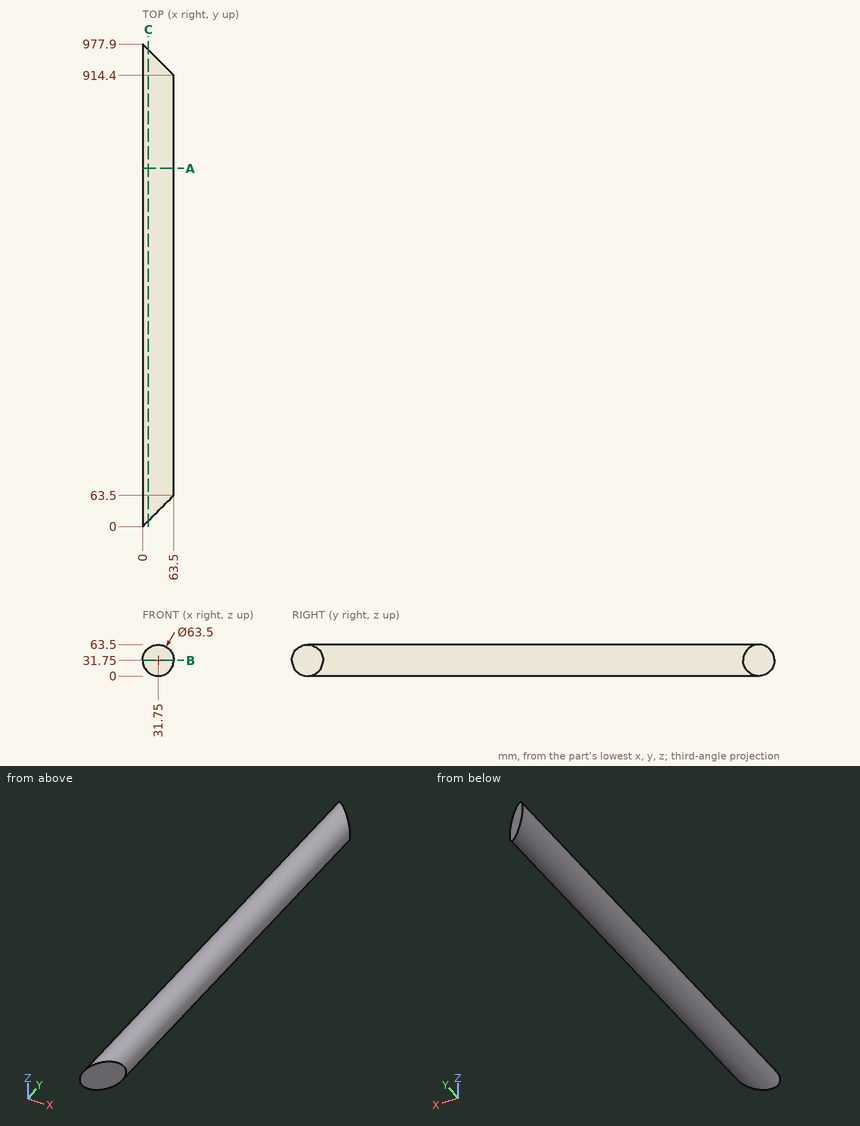
Can you work these out from the drawing? Everything is in mm from the part's minimum corner. Round coordinates to 2 decimals unless told otherwise and drop trailing zeros. Loops run counter-clockwise (first coordinate to the right, second up) from the corner with the lowest first, then second, coordinate; pieces in that order, holes last. Notation, with made-up numbers: (11, -26) - (62, -26) arc R6 ccw to (62, -19) - close; hole circle Ø7 at (75.5, -20). An arc over 180 degrees is marked (long way). One line per question, with ' | ' between items. Start each with the question number.
Q1. I want a section at C-C (x = 12). Write out the boundary of the cut face in (y, z).
Q2. I want a section at B-B (z = 31.75). Write out the boundary of the cut face in (x, y), then the cut area to 3 significant figures.
Q3. Will these pins go through, and if not, where does the flat tip stop? pin 1 (6 mm diameter, centred on x = 16, y = 178, fed in from -Z); pin 2 (8 mm diameter, centred on x = 12, y = 551, fed in from -Z); pin 3 (1 mm diameter, centred on x = 27.5, y = 336, fed in from -Z).
Q4. Please list where these lines run through material, in increasing order: line 1 (Z direction, x = 29, y = 134); line 2 (X direction, y = 721.5, z = 52); line 3 (X direction, y = 39, z = 49.5). Write a range as [from, to].
Q5. I want a section at A-A (y = 726). Write out the boundary of the cut face in (x, z), then the cut area to 3 significant figures.
Response values:
1) outline: (12, 6.89) - (965.9, 6.89) - (965.9, 56.61) - (12, 56.61) - close
2) outline: (0, 0) - (63.5, 63.5) - (63.5, 914.4) - (0, 977.9) - close | area: 58,100 mm²
3) pin 1: stops at z = 2.67 | pin 2: stops at z = 4.18 | pin 3: stops at z = 0.22
4) line 1: z = [0.12, 63.38] | line 2: x = [7.3, 56.2] | line 3: x = [5.43, 39]
5) outline: circle Ø63.5 at (31.75, 31.75) | area: 3,170 mm²
